Work out the finished part from the listing and answer in its coordinate system (mm). Face numbers are marked on the shaded views. A direction names the side the tool comes from. Coordinates: 2 decimals unless noted, no trailing zeros. Order: outer loops, then holes, each group sorted by start corner. A loop starts at its lowest first (then second) coordinate and runs counter-clockwise, first axis right, second up. Notation, with made-up numbers: M 84.5,-36 L 136.5,-36 A7 ccw 136.5,-26 Z; hole C -21,5.25 d6. An arc over 180 degrees is marked long. Use a Markdown table: item, result.
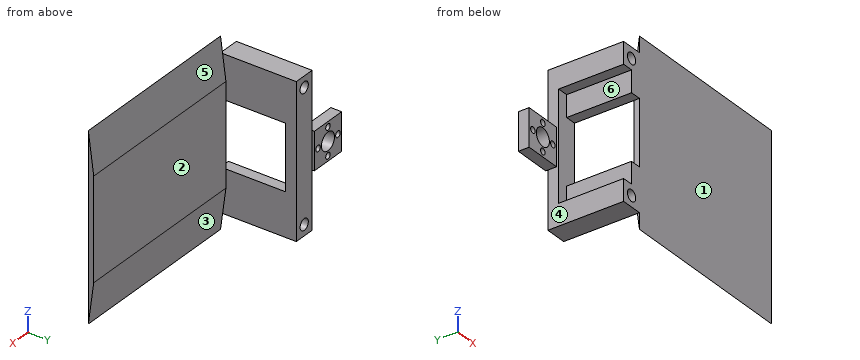
from build123d import *

# Parameters (mm, degrees)
SKETCH1_W           = 106.172
SKETCH1_H           = 107.442
BOSS_EXTRUDE1_DEPTH = 3.175
SKETCH3_W           = 12.7
SKETCH3_H           = 12.7
SKETCH3_R           = 3.302
BOSS_EXTRUDE2_DEPTH = 44.45
CUT_EXTRUDE1_DEPTH  = 106.172
SKETCH6_W           = 12.7
SKETCH6_H           = 6.35
BOSS_EXTRUDE3_DEPTH = 63.5
BOSS_EXTRUDE5_START = 1.27
SKETCH11_W          = 21.999999942
SKETCH11_H          = 21.999999942
SKETCH11_R          = 5.22699996
SKETCH11_R_2        = 1.813500056
BOSS_EXTRUDE5_DEPTH = 6.35
SKETCH12_W          = 6.35
SKETCH12_H          = 12.7
BOSS_EXTRUDE6_DEPTH = 38.1


with BuildPart() as part:
    # Sketch1 → Boss-Extrude1 (new body)
    with BuildSketch(Plane(origin=(0, 0, 0), x_dir=(1, 0, 0), z_dir=(0, 1, 0))):
        with Locations((53.086, 53.721)):
            Rectangle(SKETCH1_W, SKETCH1_H)
    extrude(amount=BOSS_EXTRUDE1_DEPTH)

    # Sketch3 → Boss-Extrude2 (add)
    # profile 1 of 2: a face of its own
    with BuildSketch(Plane(origin=(0, 0, 0), x_dir=(1, 0, 0), z_dir=(0, 1, 0))):
        with Locations((-6.35, 91.821)):
            Rectangle(SKETCH3_W, SKETCH3_H)
        with Locations(Location((-6.35, 91.821, 0), (0, 0, 270))):
            Circle(SKETCH3_R, mode=Mode.SUBTRACT)
    # profile 2 of 2: a face of its own
    with BuildSketch(Plane(origin=(0, 0, 0), x_dir=(1, 0, 0), z_dir=(0, 1, 0))):
        with Locations((-6.35, 15.621)):
            Rectangle(SKETCH3_W, SKETCH3_H)
        with Locations(Location((-6.35, 15.621, 0), (0, 0, 90))):
            Circle(SKETCH3_R, mode=Mode.SUBTRACT)
    extrude(amount=BOSS_EXTRUDE2_DEPTH)

    # Sketch4 → Cut-Extrude1 (cut)
    with BuildSketch(Plane(origin=(106.172, 0, 0), x_dir=(0, 0, -1), z_dir=(1, 0, 0))):
        Polygon((0, 0), (24.096533231, 3.175), (0, 3.175), align=None)
        Polygon((107.442, 3.175), (107.442, 0), (83.345466769, 3.175), align=None)
    extrude(amount=-CUT_EXTRUDE1_DEPTH, mode=Mode.SUBTRACT)

    # Sketch6 → Boss-Extrude3 (add)
    with BuildSketch(Plane.XY.offset(-85.471)):
        with Locations((-6.35, 41.275)):
            Rectangle(SKETCH6_W, SKETCH6_H)
    extrude(amount=BOSS_EXTRUDE3_DEPTH)

    # Sketch11 → Boss-Extrude5 (add)
    with BuildSketch(Plane(origin=(0, 44.45, 0), x_dir=(1, 0, 0), z_dir=(0, 1, 0)).offset(BOSS_EXTRUDE5_START)):
        with Locations((-23.699999971, 53.721)):
            Rectangle(SKETCH11_W, SKETCH11_H)
        with Locations(Location((-23.699999971, 53.721, 0), (0, 0, 270))):
            Circle(SKETCH11_R, mode=Mode.SUBTRACT)
        with Locations(Location((-23.699999971, 61.721000002, 0), (0, 0, 270))):
            Circle(SKETCH11_R_2, mode=Mode.SUBTRACT)
        with Locations(Location((-15.699999969, 53.721, 0), (0, 0, 270))):
            Circle(SKETCH11_R_2, mode=Mode.SUBTRACT)
        with Locations(Location((-23.699999971, 45.720999998, 0), (0, 0, 270))):
            Circle(SKETCH11_R_2, mode=Mode.SUBTRACT)
        with Locations(Location((-31.699999973, 53.721, 0), (0, 0, 270))):
            Circle(SKETCH11_R_2, mode=Mode.SUBTRACT)
    extrude(amount=-BOSS_EXTRUDE5_DEPTH)

    # Sketch12 → Boss-Extrude6 (add)
    with BuildSketch(Plane.XZ):
        with Locations((-3.175, -28.321)):
            Rectangle(SKETCH12_W, SKETCH12_H)
        with Locations((-3.175, -79.121)):
            Rectangle(SKETCH12_W, SKETCH12_H)
    extrude(amount=-BOSS_EXTRUDE6_DEPTH)


solid = part.part
1. Section D-D on z = -26 is taken. Determine the outline of the cut face in (x, y) (3 decimals).
Answers below:
| item | result |
|---|---|
| outline | M -12.7,38.1 L -6.35,38.1 L -6.35,0 L 106.172,0 L 106.172,3.175 L 0,3.175 L 0,44.45 L -12.7,44.45 Z |
2. Section C-C on z = -39.5 is taken. Determine the outline of the cut face in (x, y) (3 decimals).
Answers below:
| item | result |
|---|---|
| outline | M -12.7,38.1 L 0,38.1 L 0,44.45 L -12.7,44.45 Z; M 0,0 L 106.172,0 L 106.172,3.175 L 0,3.175 Z |
3. For a pull along Z with two mould halves and no side action, classify the marked faces 4, 5 and 6 as +Z half, -Z half, draft (parallel to the pull), parting line (faces both ways), or undercut.
Answers below:
| item | result |
|---|---|
| face 4 | draft |
| face 5 | +Z half |
| face 6 | undercut |
4. For the marked faces 1, 2 and 3, determine the directions among +Z, -Z, +X, -X, +Y, -Y from which every point of the face is accessible in a straight line to the end or side of a thin tool.
Answers below:
| item | result |
|---|---|
| face 1 | +Z, -Z, +X, -X, -Y |
| face 2 | +Z, -Z, +X, +Y |
| face 3 | -Z, +X, +Y |
5. Find the intervals of material crossed by probe 1 along Z at (x, y) = (-6, 26); probe 2 along X at (y, z) = (14.5, -15.5); probe 3 along Z at (x, y) = (-23, 43), in increasing order.
Answers below:
| item | result |
|---|---|
| probe 1 | -98.17 to -95.1, -88.54 to -72.77, -34.67 to -18.9, -12.34 to -9.27 |
| probe 2 | -12.7 to -9.65, -3.05 to 0 |
| probe 3 | -64.72 to -63.39, -60.05 to -58.9, -48.54 to -47.39, -44.05 to -42.72 |
6. Section A-A on y = 8 is taken. Determine the outline of the cut face in (x, z), then the cut area to 3 significant figures.
Answers below:
| item | result |
|---|---|
| outline | M -12.7,-98.17 L 0,-98.17 L 0,-72.77 L -6.35,-72.77 L -6.35,-85.47 L -12.7,-85.47 Z; M -12.7,-21.97 L -6.35,-21.97 L -6.35,-34.67 L 0,-34.67 L 0,-9.27 L -12.7,-9.27 Z; hole C -6.35,-91.82 d6.6; hole C -6.35,-15.62 d6.6 |
| area | 415 mm² |
7. Flat-ended cylindrical pins translate along their axes: P1, Ø6, axis at x = 16, z = -80.5, coming from the +Y side (3 decimals); P2, Ø14, axis at y = 24, z = -76.5, coming from the -X side; P3, Ø17.5, axis at x = -22.5, z = -49.5, coming from the -Y side. Find the tip coordinate at first contact, or state that the pin passes through.
Answers below:
| item | result |
|---|---|
| P1 | y = 3.175 |
| P2 | x = -6.35 |
| P3 | y = 39.37 |
8. Section B-B on x = -23.7 is taken. Determine the outline of the cut face in (y, z).
Answers below:
| item | result |
|---|---|
| outline | M 39.37,-64.72 L 45.72,-64.72 L 45.72,-63.53 L 39.37,-63.53 Z; M 39.37,-59.91 L 45.72,-59.91 L 45.72,-58.95 L 39.37,-58.95 Z; M 39.37,-48.49 L 45.72,-48.49 L 45.72,-47.53 L 39.37,-47.53 Z; M 39.37,-43.91 L 45.72,-43.91 L 45.72,-42.72 L 39.37,-42.72 Z |
